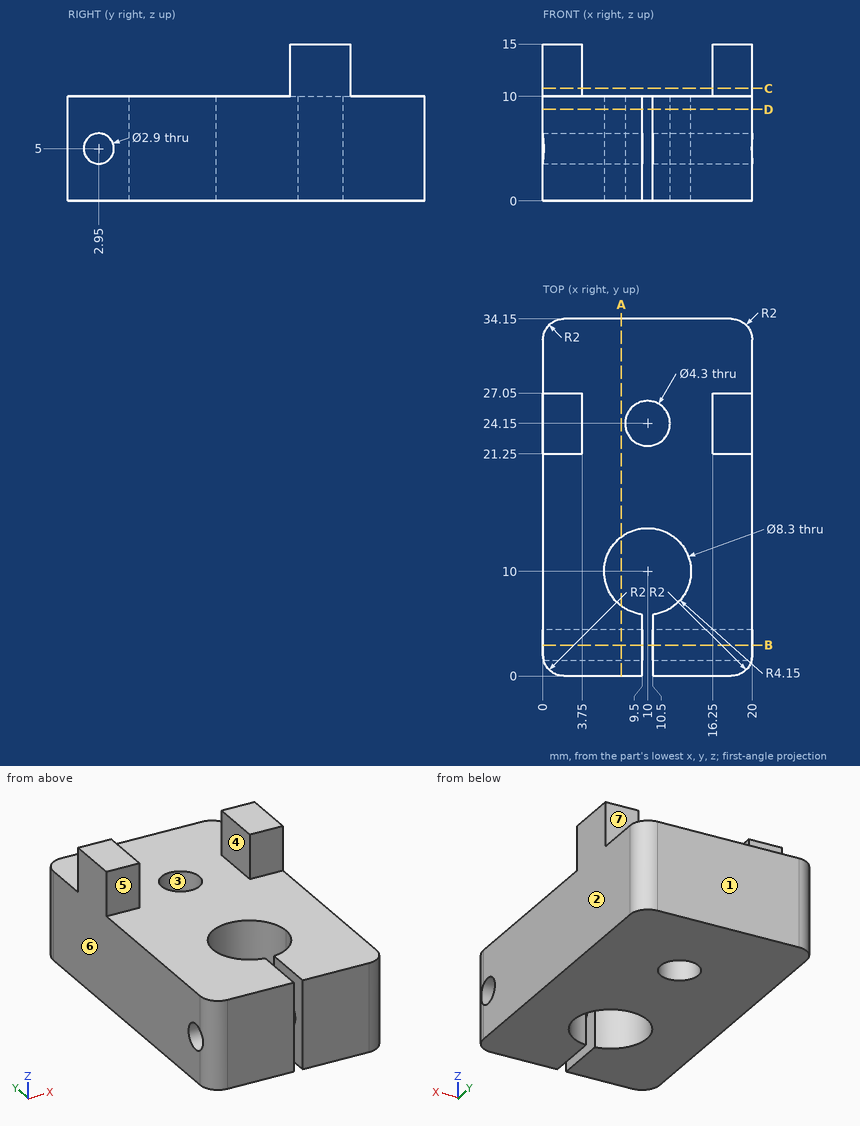
Drawing for the job (mm, zero at the part's lowest x, y, z). A direction names the side the tool comes from. Round coordinates to 2 decimals unless told otherwise and drop trailing zeros. Loops run counter-clockwise (first coordinate to the right, second up) from the corner with the lowest first, then second, coordinate; pieces in that order, holes last. Notation, with made-up numbers: M -7.5,18 L 33.5,18 A35 ccw 33.5,51 Z; hole C 33,26.5 d10. An arc over 180 degrees is marked long. Use a Markdown table: item, result. Add a question column.
(1) Drill centre lines: line 1 (Y direction, x = 10, z = 3.5); line 2 (Z direction, x = 5, y = 2.95); line 3 (Y direction, x = 11, z = 0.5). Where is each one in solid material? Low to high.
(2) Pull direction X, two halves, no side cores. Call the marked faces 1, 2, 3 and 4: +X half, -X half, draft (parallel to the pull), parting line (faces both ways), or undercut.
(3) Which spindle directions (+Z, -Z, +X, -X, +Y, -Y) get a long thin tool onto all of the face, cutting with end or side? Do the marked faces 5, 6 and 7. Say none if no direction does.
(4) Cut at C-C (z = 10.75). Give the cut face in (x, y).
(5) Cut at A-A (x = 7.5). Give the cut face in (y, z), and give its area (3 significant figures).
(6) Flat gauge pins, fed straight in: pin 1 (1.5 mm diameter, centred on x = 13.5, z = 11.5, fed in from -Y); pin 2 (1.9 mm diameter, centred on x = 1.5, z = 13, fed in from -Y); pin 3 (3 mm diameter, centred on x = 16.5, y = 14.5, fed in from +Z); pin 4 (1.1 mm diameter, centred on x = 3, z = 12.5, fed in from +Y). Where does each tip first touch, or does it go through?
(7) Cut at B-B (y = 2.95). Give the cut face in (x, z).
(8) Cut at D-D (z = 8.75). Give the cut face in (x, y), and give its area (3 significant figures).
Geometry says:
| question | item | result |
|---|---|---|
| 1 | line 1 | y = 14.15 to 22, 26.3 to 34.15 |
| 1 | line 2 | z = 0 to 3.55, 6.45 to 10 |
| 1 | line 3 | y = 0 to 5.97, 14.03 to 22.25, 26.05 to 34.15 |
| 2 | face 1 | draft |
| 2 | face 2 | +X half |
| 2 | face 3 | undercut |
| 2 | face 4 | undercut |
| 3 | face 5 | +Z, +X, -X, -Y |
| 3 | face 6 | +Z, -Z, -X, +Y, -Y |
| 3 | face 7 | +Z, +X, -X, +Y |
| 4 | outline | M 0,21.25 L 3.75,21.25 L 3.75,27.05 L 0,27.05 Z; M 16.25,21.25 L 20,21.25 L 20,27.05 L 16.25,27.05 Z |
| 5 | outline | M 0,0 L 6.69,0 L 6.69,10 L 0,10 Z; M 13.31,0 L 34.15,0 L 34.15,10 L 13.31,10 Z; hole C 2.95,5 d2.9 |
| 5 | area | 269 mm² |
| 6 | pin 1 | passes through |
| 6 | pin 2 | stops at y = 21.25 |
| 6 | pin 3 | stops at z = 10 |
| 6 | pin 4 | stops at y = 27.05 |
| 7 | outline | M 0,0 L 9.5,0 L 9.5,3.55 L 0,3.55 Z; M 0,6.45 L 9.5,6.45 L 9.5,10 L 0,10 Z; M 10.5,0 L 20,0 L 20,3.55 L 10.5,3.55 Z; M 10.5,6.45 L 20,6.45 L 20,10 L 10.5,10 Z |
| 8 | outline | M 0,2 A2 ccw 2,0 L 9.5,0 L 9.5,5.88 A4.15 cw long 10.5,5.88 L 10.5,0 L 18,0 A2 ccw 20,2 L 20,32.15 A2 ccw 18,34.15 L 2,34.15 A2 ccw 0,32.15 Z; hole C 10,24.15 d4.3 |
| 8 | area | 605 mm² |
